Model file for the job. Use its own axes, mm. A direction names the side the tool comes from. Round coordinates to 2 decimals unless told otherwise and drop trailing zeros. Write each loop counter-clockwise with the first axis right and the second up, starting at its lowest first coordinate (ties: lowest second). Pieces come first, ordered by that corner, then holes. Notation, with made-up numbers: (3, 41) - (31, 41) arc R18 cw to (31, 72) - close; hole circle Ø3 at (-28, 60.25). An arc over 180 degrees is marked (long way). Answer as a JSON object with one key per item and string values. Group by question number.
from build123d import *

# Parameters (mm, degrees)
CROQUIS1_R                = 1.5
SALIENTE_EXTRUIR1_DEPTH   = 4
CROQUIS2_R                = 2.9
CORTAR_EXTRUIR1_DEPTH     = 2
SALIENTE_EXTRUIR2_DEPTH   = 65
CORTAR_EXTRUIR2_OUTLINE_W = 7.281077338
CORTAR_EXTRUIR2_OUTLINE_H = 8.780929931
CORTAR_EXTRUIR2_DEPTH     = 8.6
CORTAR_EXTRUIR2_TAPER     = -65
CROQUIS5_W                = 41.142355125
CROQUIS5_H                = 35.377069929
CORTAR_EXTRUIR3_DEPTH     = 10
SALIENTE_EXTRUIR3_DEPTH   = 7
CORTAR_EXTRUIR4_DEPTH     = 5
CORTAR_EXTRUIR5_START     = -7
CROQUIS8_W                = 2.5
CROQUIS8_H                = 1.5
CORTAR_EXTRUIR5_DEPTH     = 7
CORTAR_EXTRUIR6_DEPTH     = 10
SALIENTE_EXTRUIR4_DEPTH   = 3.7
SALIENTE_EXTRUIR5_DEPTH   = 2.558793
CORTAR_EXTRUIR7_DEPTH     = 10
CROQUIS14_W               = 20.903204772
CROQUIS14_H               = 28.789293723
CORTAR_EXTRUIR8_DEPTH     = 10
SALIENTE_EXTRUIR6_START   = -4
CROQUIS15_R               = 1.5
SALIENTE_EXTRUIR6_DEPTH   = 4
CROQUIS16_R               = 2.9
CORTAR_EXTRUIR9_DEPTH     = 2
SALIENTE_EXTRUIR7_START   = -4
SALIENTE_EXTRUIR7_DEPTH   = 4


# Read off the part's stored shape, not the designer's step: Cortar-Extruir2
with BuildPart() as part:
    # Croquis1 → Saliente-Extruir1 (new body)
    with BuildSketch(Plane.XY):
        with BuildLine():
            Line((-55.370631899, 7.045687646), (-55.370631899, 3.345687646))
            ThreePointArc((-55.370631899, 3.345687646), (-61.070631899, -0.995420457), (-66.770631899, 3.345687646))
            Line((-66.770631899, 3.345687646), (-66.770631899, 7.045687646))
            ThreePointArc((-66.770631899, 7.045687646), (-61.070631899, 12.745687646), (-55.370631899, 7.045687646))
        make_face()
        with Locations((-61.070631899, 7.045687646)):
            Circle(CROQUIS1_R, mode=Mode.SUBTRACT)
    extrude(amount=SALIENTE_EXTRUIR1_DEPTH)

    # Croquis2 → Cortar-Extruir1 (cut)
    with BuildSketch(Plane.XY.offset(4)):
        with Locations((-61.070631899, 7.045687646)):
            Circle(CROQUIS2_R)
    extrude(amount=-CORTAR_EXTRUIR1_DEPTH, mode=Mode.SUBTRACT)

    # Croquis3 → Saliente-Extruir2 (add)
    with BuildSketch(Plane.XY.offset(4)):
        with BuildLine():
            Line((-63.970631899, 7.045687646), (-66.770631899, 7.045687646))
            Line((-66.770631899, 7.045687646), (-66.770631899, 3.345687646))
            ThreePointArc((-66.770631899, 3.345687646), (-61.070631899, -0.995420457), (-55.370631899, 3.345687646))
            Line((-55.370631899, 3.345687646), (-55.370631899, 7.045687646))
            Line((-55.370631899, 7.045687646), (-58.170631899, 7.045687646))
            ThreePointArc((-58.170631899, 7.045687646), (-61.070631899, 4.145687646), (-63.970631899, 7.045687646))
        make_face()
    extrude(amount=SALIENTE_EXTRUIR2_DEPTH)

    # Cortar-Extruir2 outline → Cortar-Extruir2 (cut)
    with BuildSketch(Plane.YZ.offset(-58.170631899)):
        with Locations((3.405148977, 64.609535034)):
            Rectangle(CORTAR_EXTRUIR2_OUTLINE_W, CORTAR_EXTRUIR2_OUTLINE_H)
    extrude(amount=-CORTAR_EXTRUIR2_DEPTH, taper=CORTAR_EXTRUIR2_TAPER, mode=Mode.SUBTRACT)

    # Croquis5 → Cortar-Extruir3 (cut)
    with BuildSketch(Plane(origin=(-70.846238664, 0, 33.03614364), x_dir=(0.422618261740701, 0, 0.9063077870366493), z_dir=(-0.9063077870366493, 1.4037441023509523e-15, 0.422618261740701))):
        with Locations((23.845262034, -3.548141358)):
            Rectangle(CROQUIS5_W, CROQUIS5_H)
    extrude(amount=CORTAR_EXTRUIR3_DEPTH, mode=Mode.SUBTRACT)

    # Croquis6 → Saliente-Extruir3 (add)
    with BuildSketch(Plane(origin=(-70.846238664, 0, 33.03614364), x_dir=(0.422618261740701, 0, 0.9063077870366493), z_dir=(-0.9063077870366493, 1.4037441023509523e-15, 0.422618261740701))):
        with BuildLine():
            Line((31.131056203, 7.045687646), (29.993040795, 7.045687646))
            add(Edge.make_bspline(
                [(16.269071612, 7.045687646), (16.269071612, 4.145687646), (23.131056203, 4.145687646), (29.993040795, 4.145687646), (29.993040795, 7.045687646)],
                knots=[3.141592654, 3.141592654, 3.141592654, 4.71238898, 4.71238898, 6.283185307, 6.283185307, 6.283185307], degree=2, weights=[1, 0.707106781, 1, 0.707106781, 1]))
            Line((16.269071612, 7.045687646), (15.131056203, 7.045687646))
            Line((15.131056203, 7.045687646), (15.131056203, -13.654312354))
            Line((15.131056203, -13.654312354), (31.131056203, -13.654312354))
            Line((31.131056203, -13.654312354), (31.131056203, 7.045687646))
        make_face()
    extrude(amount=SALIENTE_EXTRUIR3_DEPTH)

    # Croquis7 → Cortar-Extruir4 (cut)
    with BuildSketch(Plane(origin=(-77.190393173, 0, 35.994471473), x_dir=(0.42261826174070094, 0, 0.9063077870366492), z_dir=(-0.9063077870366493, 1.403744102350952e-15, 0.422618261740701))):
        with BuildLine():
            Line((25.381056203, 4.145687646), (26.731056203, -3.854312354))
            Line((26.731056203, -3.854312354), (31.131056203, -3.854312354))
            Line((31.131056203, -3.854312354), (31.131056203, -10.654312354))
            Line((31.131056203, -10.654312354), (15.131056203, -10.654312354))
            Line((15.131056203, -10.654312354), (15.131056203, -3.854312354))
            Line((15.131056203, -3.854312354), (19.531056203, -3.854312354))
            Line((19.531056203, -3.854312354), (20.881056203, 4.145687646))
            Line((20.881056203, 4.145687646), (20.881056203, 4.306015013))
            add(Edge.make_bspline(
                [(20.881056203, 4.306015013), (23.131056203, 3.97597782), (25.381056203, 4.306015013)],
                knots=[4.378316067, 4.378316067, 4.378316067, 5.046461894, 5.046461894, 5.046461894], degree=2, weights=[1, 0.944714701, 1]))
            Line((25.381056203, 4.306015013), (25.381056203, 4.145687646))
        make_face()
    extrude(amount=-CORTAR_EXTRUIR4_DEPTH, mode=Mode.SUBTRACT)

    # Croquis8 → Cortar-Extruir5 (cut)
    with BuildSketch(Plane(origin=(-77.190393173, 0, 35.994471473), x_dir=(0.42261826174070094, 0, 0.9063077870366492), z_dir=(-0.9063077870366493, 1.403744102350952e-15, 0.422618261740701)).offset(CORTAR_EXTRUIR5_START)):
        with Locations((17.381056203, -2.104312354)):
            Rectangle(CROQUIS8_W, CROQUIS8_H)
        with Locations((28.881056203, -2.104312354)):
            Rectangle(CROQUIS8_W, CROQUIS8_H)
    extrude(amount=CORTAR_EXTRUIR5_DEPTH, mode=Mode.SUBTRACT)

    # Croquis9 → Cortar-Extruir6 (cut)
    with BuildSketch(Plane(origin=(0, 7.045687646, 0), x_dir=(1, 0, 0), z_dir=(0, 1, 0))):
        Polygon((-57.689685805, -61.250462296), (-55.370631899, -60.1690697), (-55.370631899, -66.223689447), align=None)
    extrude(amount=-CORTAR_EXTRUIR6_DEPTH, mode=Mode.SUBTRACT)

    # Croquis10 → Saliente-Extruir4 (add)
    with BuildSketch(Plane(origin=(0, 7.045687646, 0), x_dir=(1, 0, 0), z_dir=(0, 1, 0))):
        Polygon((-66.770631899, -41.776310553), (-66.770631899, -47.8309303), (-64.451577993, -46.749537704), align=None)
    extrude(amount=-SALIENTE_EXTRUIR4_DEPTH)

    # Croquis12 → Saliente-Extruir5 (add)
    with BuildSketch(Plane(origin=(-70.846238664, 0, 33.03614364), x_dir=(0.422618261740701, 0, 0.9063077870366493), z_dir=(-0.9063077870366493, 1.4037441023509523e-15, 0.422618261740701))):
        with BuildLine():
            Line((15.131056203, 3.345687646), (15.131056203, 0.066589345))
            ThreePointArc((15.131056203, 0.066589345), (12.129139109, 1.273987016), (9.64370718, 3.345687646))
            Line((9.64370718, 3.345687646), (15.131056203, 3.345687646))
        make_face()
    extrude(amount=SALIENTE_EXTRUIR5_DEPTH)

    # Croquis13 → Cortar-Extruir7 (cut)
    with BuildSketch(Plane(origin=(0, 3.345687646, 0), x_dir=(1, 0, 0), z_dir=(0, 1, 0))):
        Polygon((-66.770631899, -47.8309303), (-66.770631899, -41.776310553), (-69.089685805, -42.857703149), align=None)
    extrude(amount=-CORTAR_EXTRUIR7_DEPTH, mode=Mode.SUBTRACT)

    # Croquis14 → Cortar-Extruir8 (cut)
    with BuildSketch(Plane(origin=(0, 0, 0), x_dir=(-1, 0, 0), z_dir=(0, 0, -1))):
        with Locations((60.961327713, 6.880035774)):
            Rectangle(CROQUIS14_W, CROQUIS14_H)
    extrude(amount=-CORTAR_EXTRUIR8_DEPTH, mode=Mode.SUBTRACT)

    # Croquis15 → Saliente-Extruir6 (add)
    with BuildSketch(Plane(origin=(0, 0, 10), x_dir=(-1, 0, 0), z_dir=(0, 0, -1)).offset(SALIENTE_EXTRUIR6_START)):
        with BuildLine():
            ThreePointArc((55.370631899, 7.045687646), (61.070631899, 12.745687646), (66.770631899, 7.045687646))
            Line((66.770631899, 7.045687646), (63.970631899, 7.045687646))
            ThreePointArc((63.970631899, 7.045687646), (61.070631899, 4.145687646), (58.170631899, 7.045687646))
            Line((58.170631899, 7.045687646), (55.370631899, 7.045687646))
        make_face()
        with Locations((61.070631899, 7.045687646)):
            Circle(CROQUIS15_R, mode=Mode.SUBTRACT)
    extrude(amount=SALIENTE_EXTRUIR6_DEPTH)

    # Croquis16 → Cortar-Extruir9 (cut)
    with BuildSketch(Plane.XY.offset(14)):
        with Locations((-61.070631899, 7.045687646)):
            Circle(CROQUIS16_R)
    extrude(amount=-CORTAR_EXTRUIR9_DEPTH, mode=Mode.SUBTRACT)

    # Croquis17 → Saliente-Extruir7 (add)
    with BuildSketch(Plane(origin=(0, 0, 10), x_dir=(-1, 0, 0), z_dir=(0, 0, -1)).offset(SALIENTE_EXTRUIR7_START)):
        with BuildLine():
            Line((55.370631899, 3.345687646), (53.370631899, 3.345687646))
            Line((53.370631899, 3.345687646), (53.370631899, 7.045687646))
            ThreePointArc((53.370631899, 7.045687646), (61.070631899, 14.745687646), (68.770631899, 7.045687646))
            Line((68.770631899, 7.045687646), (68.770631899, 3.345687646))
            Line((68.770631899, 3.345687646), (66.770631899, 3.345687646))
            Line((66.770631899, 3.345687646), (66.770631899, 7.045687646))
            ThreePointArc((66.770631899, 7.045687646), (61.070631899, 12.745687646), (55.370631899, 7.045687646))
            Line((55.370631899, 7.045687646), (55.370631899, 3.345687646))
        make_face()
    extrude(amount=SALIENTE_EXTRUIR7_DEPTH)


solid = part.part
(1) Flat gauge pins, fed straight in: pin 1 (2 mm diameter, centred on x = -67.5, z = 12, fed in from -Y); pin 2 (1.6 mm diameter, centred on x = -60, z = 59.5, fed in from +Y); pin 3 (1 mm diameter, centred on x = -55.5, z = 42, fed in from -Y); pin 4 (3 mm diameter, centred on y = 9.5, z = 36, fed in from +X). Where does each tip first touch, or does it go through?
(2) Pull direction X, two halves, no side cores. Call faces 1 (the cylindrical face through (-59.572, 7.112, 11.014)), 2 (the flat face through (-64.996, 1.672, 62.146)), 3 (the flat face through (-62, -1.354, 61)), 4 (the flat face through (-63, -3.854, 61)): pulls with the +X half, pulls with the -X half, needs draft (parallel to the pull), parting line crosses it, or undercut.
(3) Slice it at D-D (y = 12.75). Write the cut outline in (x, z).
(4) 3-axis set-ups, long thin cutter, end or side, ignore diameter. For faces 5 (the flat face through (-67, -2.854, 50)), 6 (the flat face through (-66.771, 5, 31)), 7 (the flat face through (-66, 7.046, 32)), 8 (the flat face through (-68, 3.346, 12)): which of +Z, -Z, +X, -X, +Y, -Y reach the whole face in a straight line?
(5) Slice it at C-C (y = -10). Write the cut outline in (x, z).
(6) Slice it at A-A (z = 40). Write the cut outline in (x, y), then the cut area to 3 significant figures.
(7) Drill centre lines: line 1 (Z direction, x = -62, y = -2.5); line 2 (Y direction, x = -58.75, z = 61.5); line 3 (X direction, y = 6.5, z = 17). Where is each one in solid material? Low to high. Write a range as from..to.
(8) Slice it at B-B (x = -60.5). Count the separate pieces of the cut face and the enclosed holes in it, then the cut area to 3 significant figures.
Answer:
{
 "1": {"pin 1": "y = 2.58", "pin 2": "y = 5.84", "pin 3": "y = 1.88", "pin 4": "through"},
 "2": {"face 1": "undercut", "face 2": "pulls with the -X half", "face 3": "undercut", "face 4": "needs draft"},
 "3": {"outline": "(-66.24, 10) - (-55.9, 10) - (-55.9, 14) - (-66.24, 14) - close"},
 "4": {"face 5": "none", "face 6": "-X, +Y, -Y", "face 7": "+Z, +X, -X, +Y", "face 8": "-Z, -X, -Y"},
 "5": {"outline": "(-66.26, 47.59) - (-64.45, 46.75) - (-57.69, 61.25) - (-59.5, 62.1) - close"},
 "6": {"outline": "(-66.77, 3.35) arc R5.91 ccw to (-55.37, 3.35) - (-55.37, 7.05) - (-58.17, 7.05) arc R2.9 cw to (-63.97, 7.05) - (-66.77, 7.05) - close", "area": "65.5 mm²"},
 "7": {"line 1": "52.01..56.74, 58.15..59.4, 62.16..63.26", "line 2": "-13.65..7.05", "line 3": "-66.77..-63.92, -58.22..-55.37"},
 "8": {"separate pieces": "2", "enclosed holes": "1", "area": "376 mm²"}
}
